Geometry check sheet. Reference: the model listing, model coordinates, mm. Face numbers are marked on the shaded views. Round coordinates to 2 decimals unless told otherwise and drop trailing zeros. Write each loop counter-clockwise with the first axis right and the second up, starting at its lowest first coordinate (ties: lowest second). Pieces come first, ordered by that corner, then holes. Notation, with made-up numbers: (75.25, -32) - (106.25, -32) arc R28 ccw to (106.25, -5) - close; hole circle Ø9 at (77.5, -34). An arc over 180 degrees is marked (long way). Return JSON: item names as keys, results as strings.
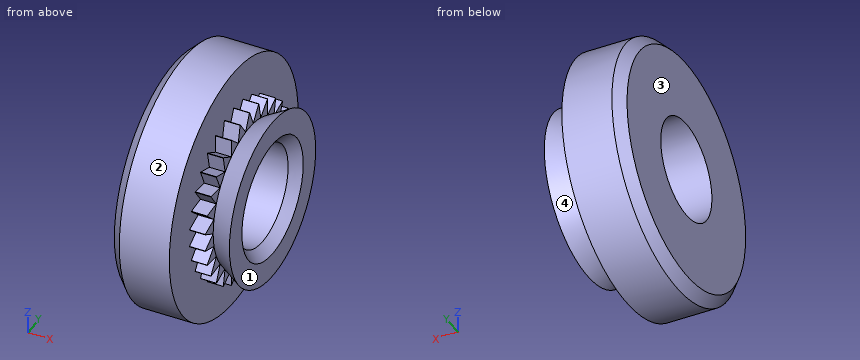
```python
from build123d import *

# Parameters (mm, degrees)
CUT_EXTRUDE_1_DEPTH      = 0.393521224
PATTERN_START            = 1.5
PATTERN_CIRCULAR_1_DEPTH = 0.393521224
HOLE_WIZARD_M31_D        = 2.5
HOLE_WIZARD_M31_DEPTH    = 8.5
HOLE_WIZARD_M31_TIP      = 0.751075774
CHAMFER_3_SIZE           = 0.25
CHAMFER_4_SIZE           = 0.25


# Read off the part's stored shape, not the designer's step: Круговой массив1
with BuildPart() as part:
    # Эскиз1 → Повернуть1 (revolve)
    with BuildSketch(Plane.XY, mode=Mode.PRIVATE) as revolve_1_sk:
        Polygon((0, 0), (0, 3.15), (1.5, 3.15), (1.5, 2.177572634), (1.893521224, 2.177572634), (1.893521224, 1.777572634), (2.469302313, 2.11), (2.469302313, 0), align=None)
    revolve(revolve_1_sk.sketch.rotate(Axis((0, 0, 0), (1, 0, 0)), 180), axis=Axis((0, 0, 0), (1, 0, 0)))

    # Эскиз2 → Вырез-Вытянуть1 (cut)
    with BuildSketch(Plane(origin=(1.893521224, 0, 0), x_dir=(0, 0, -1), z_dir=(1, 0, 0))):
        with BuildLine():
            Line((0, 1.78), (-0.222932839, 2.166131003))
            ThreePointArc((-0.222932839, 2.166131003), (0, 2.177572634), (0.222932839, 2.166131003))
            Line((0.222932839, 2.166131003), (0, 1.78))
        make_face()
    extrude(amount=-CUT_EXTRUDE_1_DEPTH, mode=Mode.SUBTRACT)

    # Круговой массив1 outline → Круговой массив1 (cut)
    with BuildSketch(Plane.YZ.offset(PATTERN_START)):
        with BuildLine():
            Line((-0.89, -1.987390896), (-0.89, -1.541525219))
            Line((-0.89, -1.541525219), (-1.276131004, -1.764458058))
            ThreePointArc((-1.276131004, -1.764458058), (-1.088786317, -1.885833219), (-0.89, -1.987390896))
        make_face()
        with BuildLine():
            Line((1.741102729, -0.37008281), (2.0724455, -0.668425181))
            ThreePointArc((2.0724455, -0.668425181), (2.129987447, -0.452742808), (2.165146187, -0.232302738))
            Line((2.165146187, -0.232302738), (1.741102729, -0.37008281))
        make_face()
        with BuildLine():
            Line((1.626110915, -0.723991225), (1.888184184, -1.084704135))
            ThreePointArc((1.888184184, -1.084704135), (1.989311588, -0.885698583), (2.069534093, -0.677385571))
            Line((2.069534093, -0.677385571), (1.626110915, -0.723991225))
        make_face()
        with BuildLine():
            Line((1.44005025, -1.046257749), (1.621400159, -1.453576313))
            ThreePointArc((1.621400159, -1.453576313), (1.761693267, -1.279945079), (1.883473429, -1.092863403))
            Line((1.883473429, -1.092863403), (1.44005025, -1.046257749))
        make_face()
        with BuildLine():
            Line((1.191052479, -1.322797789), (1.283753166, -1.758920232))
            ThreePointArc((1.283753166, -1.758920232), (1.457080496, -1.618251835), (1.615095937, -1.460577861))
            Line((1.615095937, -1.460577861), (1.191052479, -1.322797789))
        make_face()
        with BuildLine():
            Line((0.89, -1.541525219), (0.89, -1.987390896))
            ThreePointArc((0.89, -1.987390896), (1.088786317, -1.885833219), (1.276131003, -1.764458057))
            Line((1.276131003, -1.764458057), (0.89, -1.541525219))
        make_face()
        with BuildLine():
            Line((0.55005025, -1.692880599), (0.457349563, -2.129003042))
            ThreePointArc((0.457349563, -2.129003042), (0.67290695, -2.070994643), (0.881393021, -1.99122297))
            Line((0.881393021, -1.99122297), (0.55005025, -1.692880599))
        make_face()
        with BuildLine():
            Line((0.186060665, -1.770248974), (0.004710756, -2.177567538))
            ThreePointArc((0.004710756, -2.177567538), (0.227618321, -2.165643663), (0.448133934, -2.130961884))
            Line((0.448133934, -2.130961884), (0.186060665, -1.770248974))
        make_face()
        with BuildLine():
            Line((-0.186060665, -1.770248974), (-0.448133934, -2.130961884))
            ThreePointArc((-0.448133934, -2.130961884), (-0.227618321, -2.165643663), (-0.004710756, -2.177567538))
            Line((-0.004710756, -2.177567538), (-0.186060665, -1.770248974))
        make_face()
        with BuildLine():
            Line((-0.55005025, -1.692880599), (-0.881393021, -1.99122297))
            ThreePointArc((-0.881393021, -1.99122297), (-0.67290695, -2.070994643), (-0.457349563, -2.129003042))
            Line((-0.457349563, -2.129003042), (-0.55005025, -1.692880599))
        make_face()
        with BuildLine():
            ThreePointArc((2.165146187, 0.232302738), (2.129987447, 0.452742808), (2.0724455, 0.668425181))
            Line((2.0724455, 0.668425181), (1.741102729, 0.37008281))
            Line((1.741102729, 0.37008281), (2.165146187, 0.232302738))
        make_face()
        with BuildLine():
            ThreePointArc((2.069534093, 0.677385571), (1.989311588, 0.885698583), (1.888184184, 1.084704135))
            Line((1.888184184, 1.084704135), (1.626110915, 0.723991225))
            Line((1.626110915, 0.723991225), (2.069534093, 0.677385571))
        make_face()
        with BuildLine():
            ThreePointArc((1.883473429, 1.092863403), (1.761693267, 1.279945079), (1.621400159, 1.453576313))
            Line((1.621400159, 1.453576313), (1.44005025, 1.046257749))
            Line((1.44005025, 1.046257749), (1.883473429, 1.092863403))
        make_face()
        with BuildLine():
            ThreePointArc((1.615095937, 1.460577861), (1.457080496, 1.618251835), (1.283753166, 1.758920232))
            Line((1.283753166, 1.758920232), (1.191052479, 1.322797789))
            Line((1.191052479, 1.322797789), (1.615095937, 1.460577861))
        make_face()
        with BuildLine():
            ThreePointArc((1.276131003, 1.764458057), (1.088786317, 1.885833219), (0.89, 1.987390896))
            Line((0.89, 1.987390896), (0.89, 1.541525219))
            Line((0.89, 1.541525219), (1.276131003, 1.764458057))
        make_face()
        with BuildLine():
            ThreePointArc((0.881393021, 1.99122297), (0.67290695, 2.070994643), (0.457349563, 2.129003042))
            Line((0.457349563, 2.129003042), (0.55005025, 1.692880599))
            Line((0.55005025, 1.692880599), (0.881393021, 1.99122297))
        make_face()
        with BuildLine():
            ThreePointArc((0.448133934, 2.130961884), (0.227618321, 2.165643663), (0.004710756, 2.177567538))
            Line((0.004710756, 2.177567538), (0.186060665, 1.770248974))
            Line((0.186060665, 1.770248974), (0.448133934, 2.130961884))
        make_face()
        with BuildLine():
            ThreePointArc((-0.004710756, 2.177567538), (-0.227618321, 2.165643663), (-0.448133934, 2.130961884))
            Line((-0.448133934, 2.130961884), (-0.186060665, 1.770248974))
            Line((-0.186060665, 1.770248974), (-0.004710756, 2.177567538))
        make_face()
        with BuildLine():
            ThreePointArc((-0.457349563, 2.129003042), (-0.67290695, 2.070994643), (-0.881393021, 1.99122297))
            Line((-0.881393021, 1.99122297), (-0.55005025, 1.692880599))
            Line((-0.55005025, 1.692880599), (-0.457349563, 2.129003042))
        make_face()
        with BuildLine():
            ThreePointArc((-0.89, 1.987390896), (-1.088786317, 1.885833219), (-1.276131004, 1.764458058))
            Line((-1.276131004, 1.764458058), (-0.89, 1.541525219))
            Line((-0.89, 1.541525219), (-0.89, 1.987390896))
        make_face()
        with BuildLine():
            ThreePointArc((-1.283753166, 1.758920232), (-1.457080497, 1.618251835), (-1.615095937, 1.460577861))
            Line((-1.615095937, 1.460577861), (-1.191052479, 1.322797789))
            Line((-1.191052479, 1.322797789), (-1.283753166, 1.758920232))
        make_face()
        with BuildLine():
            ThreePointArc((-1.621400159, 1.453576313), (-1.761693268, 1.27994508), (-1.883473429, 1.092863403))
            Line((-1.883473429, 1.092863403), (-1.44005025, 1.046257749))
            Line((-1.44005025, 1.046257749), (-1.621400159, 1.453576313))
        make_face()
        with BuildLine():
            ThreePointArc((-1.888184185, 1.084704135), (-1.989311588, 0.885698583), (-2.069534094, 0.677385571))
            Line((-2.069534094, 0.677385571), (-1.626110915, 0.723991225))
            Line((-1.626110915, 0.723991225), (-1.888184185, 1.084704135))
        make_face()
        with BuildLine():
            ThreePointArc((-2.072445501, 0.668425181), (-2.129987447, 0.452742808), (-2.165146188, 0.232302738))
            Line((-2.165146188, 0.232302738), (-1.741102729, 0.37008281))
            Line((-1.741102729, 0.37008281), (-2.072445501, 0.668425181))
        make_face()
        with BuildLine():
            ThreePointArc((-2.166131004, 0.222932839), (-2.177572634, 0), (-2.166131004, -0.222932839))
            Line((-2.166131004, -0.222932839), (-1.78, 0))
            Line((-1.78, 0), (-2.166131004, 0.222932839))
        make_face()
        with BuildLine():
            ThreePointArc((-2.165146188, -0.232302738), (-2.129987447, -0.452742808), (-2.072445501, -0.668425181))
            Line((-2.072445501, -0.668425181), (-1.741102729, -0.37008281))
            Line((-1.741102729, -0.37008281), (-2.165146188, -0.232302738))
        make_face()
        with BuildLine():
            ThreePointArc((-2.069534094, -0.677385571), (-1.989311588, -0.885698583), (-1.888184185, -1.084704135))
            Line((-1.888184185, -1.084704135), (-1.626110915, -0.723991225))
            Line((-1.626110915, -0.723991225), (-2.069534094, -0.677385571))
        make_face()
        with BuildLine():
            ThreePointArc((-1.883473429, -1.092863403), (-1.761693268, -1.27994508), (-1.621400159, -1.453576313))
            Line((-1.621400159, -1.453576313), (-1.44005025, -1.046257749))
            Line((-1.44005025, -1.046257749), (-1.883473429, -1.092863403))
        make_face()
        with BuildLine():
            ThreePointArc((-1.615095937, -1.460577861), (-1.457080497, -1.618251835), (-1.283753166, -1.758920232))
            Line((-1.283753166, -1.758920232), (-1.191052479, -1.322797789))
            Line((-1.191052479, -1.322797789), (-1.615095937, -1.460577861))
        make_face()
    extrude(amount=PATTERN_CIRCULAR_1_DEPTH, mode=Mode.SUBTRACT)

    # Отверстие обработанное метчиком M31
    with Locations(Plane.ZY):
        with Locations((0, 0)):
            Hole(HOLE_WIZARD_M31_D / 2, depth=HOLE_WIZARD_M31_DEPTH)
            with Locations((0, 0, -(HOLE_WIZARD_M31_DEPTH + HOLE_WIZARD_M31_TIP / 2))):  # 118° drill point
                Cone(0, HOLE_WIZARD_M31_D / 2, HOLE_WIZARD_M31_TIP, mode=Mode.SUBTRACT)

    # Фаска3
    chamfer_3_edges = [part.edges().sort_by_distance(p)[0] for p in [
        (2.469302313, 0, 1.25),
    ]]
    chamfer(chamfer_3_edges, length=CHAMFER_3_SIZE)

    # Фаска4
    chamfer_4_edges = [part.edges().sort_by_distance(p)[0] for p in [
        (0, 3.15, 0),
    ]]
    chamfer(chamfer_4_edges, length=CHAMFER_4_SIZE)


solid = part.part
```
(1) Gauge pin test, flat end, axial feed: pin 1 (1.5 mm diameter, centred on y = 0, z = 0, fed in from +X). Record the tip position at first contact, or that the pin passes through.
Response values:
{"pin 1": "passes through"}
(2) Section check A-A, the plane x = 0.5. Enter the section's corners in (y, z).
Response values:
{"outline": "circle Ø6.3 at (0, 0); hole circle Ø2.5 at (0, 0)"}
(3) Release check for a two-part mould opening along X. For the marked faces 1, 2, 3 and 4 record: pulls with the +X half, pulls with the -X half, needs draft (parallel to the pull), parting line crosses it, or undercut.
Response values:
{"face 1": "pulls with the +X half", "face 2": "needs draft", "face 3": "pulls with the -X half", "face 4": "undercut"}
(4) Section check B-B, the plane x = 2.3. Enter the section's corners in (y, z), plus the area to 3 significant figures.
Response values:
{"outline": "circle Ø4.02 at (0, 0); hole circle Ø2.66 at (0, 0)", "area": "7.16 mm^2"}
(5) Material ranges on line 1 along X through (y, z) = (-2, -0.25); line 2 along X through (y, z) = (0, -2.5); line 3 along Z through (x, y) = (1.7, 0.25), recorded low to high. Write a range as [from, to].
Response values:
{"line 1": "x = [0, 1.89], [2.31, 2.47]", "line 2": "x = [0, 1.5]", "line 3": "z = [-1.86, -1.22], [1.22, 1.86]"}
